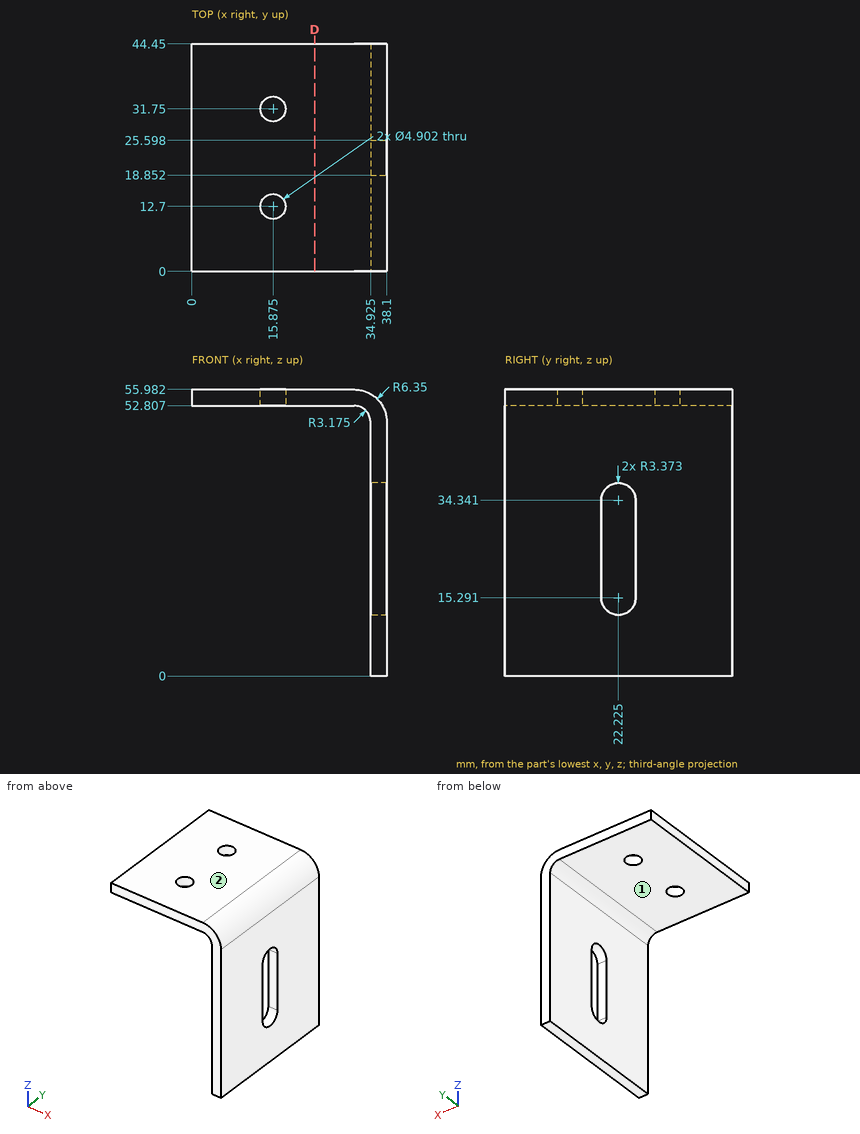
For this review, use the dimensioned drawing (mm, ordinates from the lowest corner) and the shaded views. A direction names the side the tool comes from. Give positions to 0.01 mm unless a question says otherwise; leave off trailing zeros. Order: outer loops, then holes, each group sorted by start corner. A loop starts at its lowest first (then second) coordinate and runs counter-clockwise, first axis right, second up. Notation, with made-up numbers: (71, -20.75) - (119, -20.75) arc R26 cw to (119, -2.75) - close; hole circle Ø6 at (88, -24.75). An arc over 180 degrees is marked (long way). Use a Markdown table: item, result. Add a question column.
(1) Machinability: for the marked faces 1 and 2, which of the approach directions +Z, -Z, +X, -X, +Y, -Y give a long, thin tool a straight path to every point of the face, cutting with its end or side? Answer none if there is none.
(2) Clearance check with flat-ended pins moving along their axes: P1, Ø6, axis at y = 15.5, z = 22, coming from the -X side (3 decimals); P2, Ø3, axis at x = 15.875, y = 31.75, coming from the +Z side; P3, Ø3, axis at y = 34.5, z = 49.5, coming from the -X side (1 decimal); P4, Ø6.5, axis at x = 15.875, y = 12.7, coming from the -Z side. State where each tip first meets the part, or that it passes through.
(3) Add section D-D on x = 24. Give the boundary of the cut face in (y, z).
(4) Wall thickness on probe 1 along Z at (x, y) = (29, 34.5); probe 2 along X at (y, z) = (15, 31) (1 decimal); probe 3 along Y at (x, z) = (35, 23.5): over which ranges is each line inside the solid? List them lowest first. Write a range as [from, to].
Report:
| question | item | result |
|---|---|---|
| 1 | face 1 | -Z, -X, +Y, -Y |
| 1 | face 2 | +Z, +X, -X, +Y, -Y |
| 2 | P1 | stops at x = 34.925 |
| 2 | P2 | passes through |
| 2 | P3 | stops at x = 34.6 |
| 2 | P4 | stops at z = 52.81 |
| 3 | outline | (0, 52.81) - (44.45, 52.81) - (44.45, 55.98) - (0, 55.98) - close |
| 4 | probe 1 | z = [52.81, 55.98] |
| 4 | probe 2 | x = [34.9, 38.1] |
| 4 | probe 3 | y = [0, 18.85], [25.6, 44.45] |
